For this review, use the dimensioned drawing (mm, ordinates from the lowest corner) and the shaded views. Give positions to 0.01 mm unless a question says otherwise; leave off trailing zeros. Write each loop counter-clockwise with the first axis right and the second up, starting at its lowest first coordinate (ties: lowest second). Pieces come first, ordered by that corner, then holes.
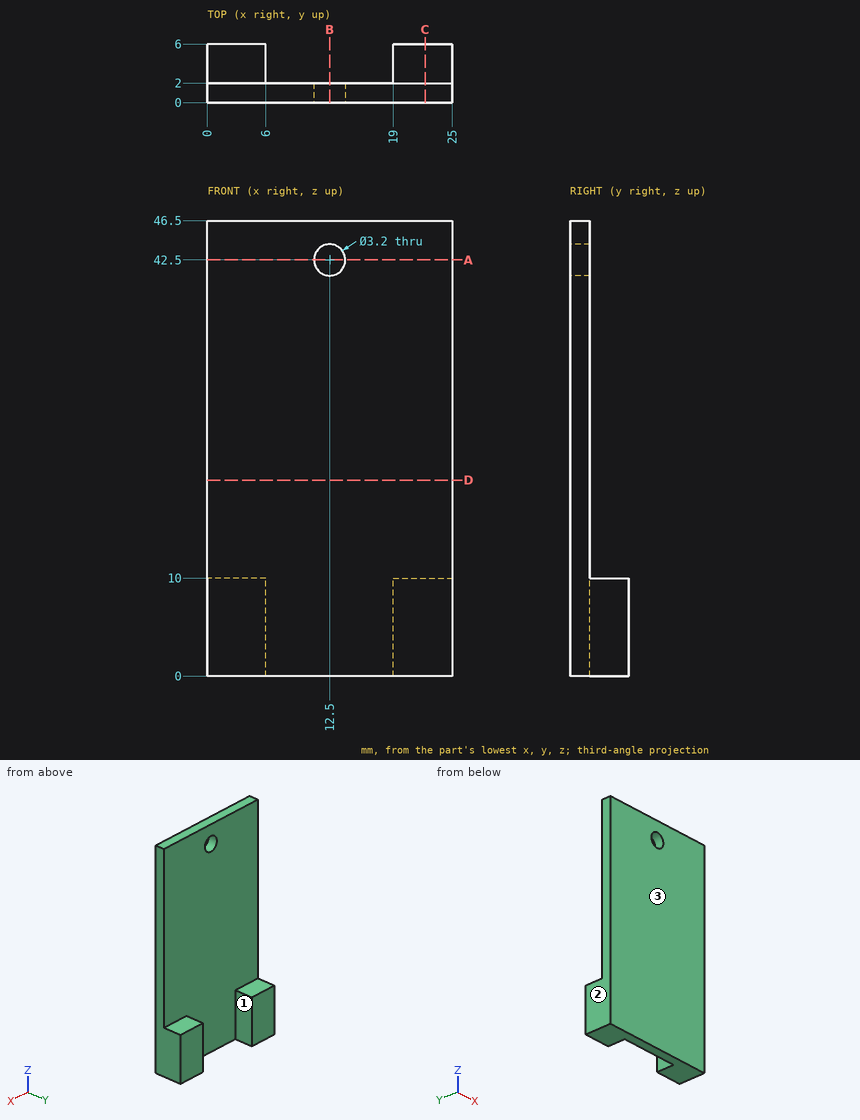
(1) For L1, parallel to Z at x = 12.5, y = 1; L2, parallel to X at y = 0.65, z = 42.5; L3, parallel to X at y = 4.45, z = 9, list the stretches that pass through material, from the lowest coordinate up.
(2) We need section B-B (x = 12.5). Write out the cut boundary in (y, z).
(3) We need section A-A (z = 42.5). Write out the cut boundary in (x, y), and give its area (3 significant figures).
(4) We need section D-D (z = 20). Write out the cut boundary in (x, y).
(5) The part is to be moulded in two halves that separate along X. For the marked faces 1, 2 and 3, say which applies: +X half, -X half, draft (parallel to the pull), parting line (faces both ways), or undercut.
(6) We need section C-C (x = 22.25). Write out the cut boundary in (y, z).
(7) Clearance check with flat-ended pins moving along their axes: pin 1 Ø2 at (x, y) = (21, 4.5) entering from +Z; pin 2 Ø4 at (x, z) = (16.5, 21.5) entering from +Y. State where each tip first meets the part, or that it passes through.
The answers:
1. L1: z = 0 to 40.9, 44.1 to 46.5
1. L2: x = 0 to 10.9, 14.1 to 25
1. L3: x = 0 to 6, 19 to 25
2. outline: (0, 0) - (2, 0) - (2, 40.9) - (0, 40.9) - close; (0, 44.1) - (2, 44.1) - (2, 46.5) - (0, 46.5) - close
3. outline: (0, 0) - (10.9, 0) - (10.9, 2) - (0, 2) - close; (14.1, 0) - (25, 0) - (25, 2) - (14.1, 2) - close
3. area: 43.6 mm2
4. outline: (0, 0) - (25, 0) - (25, 2) - (0, 2) - close
5. face 1: undercut
5. face 2: -X half
5. face 3: draft
6. outline: (0, 0) - (6, 0) - (6, 10) - (2, 10) - (2, 46.5) - (0, 46.5) - close
7. pin 1: stops at z = 10
7. pin 2: stops at y = 2
